from build123d import *

# Parameters (mm, degrees)
BOSS_EXTRUDE1_DEPTH = 6
SKETCH3_R           = 2
CUT_EXTRUDE1_DEPTH  = 5


with BuildPart() as part:
    # Sketch1 → Boss-Extrude1 (new body)
    with BuildSketch(Plane(origin=(0, 0, 0), x_dir=(1, 0, 0), z_dir=(0, 1, 0))):
        with BuildLine():
            Line((-1, 2.291287847), (-1, 4.291287847))
            Line((-1, 4.291287847), (1, 4.291287847))
            Line((1, 4.291287847), (1, 2.291287847))
            ThreePointArc((1, 2.291287847), (2.5, 0), (1, -2.291287847))
            Line((1, -2.291287847), (1, -4.291287847))
            Line((1, -4.291287847), (-1, -4.291287847))
            Line((-1, -4.291287847), (-1, -2.291287847))
            ThreePointArc((-1, -2.291287847), (-2.5, 0), (-1, 2.291287847))
        make_face()
    extrude(amount=BOSS_EXTRUDE1_DEPTH)

    # Sketch3 → Cut-Extrude1 (cut)
    with BuildSketch(Plane.XZ):
        with Locations(Location((0, 0, 0), (0, 0, 270))):
            Circle(SKETCH3_R)
    extrude(amount=-CUT_EXTRUDE1_DEPTH, mode=Mode.SUBTRACT)


solid = part.part
The model under review builds one solid part; all positions refer to its coordinate system, in mm. A direction names the side the tool comes from. Give positions to 0.01 mm unless a question says otherwise; leave off trailing zeros. Loops run counter-clockwise (first coordinate to the right, second up) from the corner with the lowest first, then second, coordinate; pieces in that order, holes last. Notation, with made-up numbers: (38, -5) -> (90, -5) arc R22 cw to (90, 21) -> close; hole circle Ø10 at (-24, 26). An arc over 180 degrees is marked (long way). Answer as a JSON object with one key per item and string values. Group by question number.
Q1. Insertion check: pin 1 (0.6 mm diameter, centred on y = 2.5, z = 3, fed in from -X); pin 2 (2 mm diameter, centred on y = 1, z = 2, fed in from -X); pin 3 (1.6 mm diameter, centred on y = 3, z = 3, fed in from +X). Each pin has a flat end and moves straight along its axis. Give the tip position at first contact, or say it passes through.
Q2. Wall thickness on line 1 along Y through (x, z) = (1.1, 1); line 2 along X through (y, z) = (4.75, 0.25); line 3 along X through (y, z) = (4.6, -1.5): over which ranges is each line inside the solid? List them lowest first.
Q3. Take a section at A-A (y = 3.8). Write out the cut boundary in (x, z), plus the area to 3 significant figures.
Q4. Tool access review of faces 1 (the flat face through (1, 3, 3)), 2 (the flat face through (-1, 3, 3)), 3 (the flat face through (-1, 3, -3)): name each direction out of +Z, -Z, +X, -X, +Y, -Y from which nothing blocks a thin tool from reaching the whole face with its end or side.
Q5. Draft analysis for pull direction Z (two halves, no side actions). For faces 4 (the flat face through (0, 5, 0)), 5 (the flat face through (0, 3, -4.291)), 6 (the flat face through (0, 6, 0)), 7 (the cylindrical face through (-2, 2, 0)), state which applies: pulls with the +Z half, pulls with the -Z half, needs draft (parallel to the pull), parting line crosses it, or undercut.
Q6. Take a section at C-C (x = 1.55). Write out the cut boundary in (y, z), plus the area to 3 significant figures.
Q7. Take a section at B-B (z = 0). Write out the cut boundary in (x, y), plus the area to 3 significant figures.
Q8. Take a section at D-D (z = 3). Write out the cut boundary in (x, y).
Answer below:
{
 "1": {"pin 1": "stops at x = -1", "pin 2": "stops at x = -2.29", "pin 3": "stops at x = 1.19"},
 "2": {"line 1": "y = 5 to 6", "line 2": "x = -2.49 to -1.98, 1.98 to 2.49", "line 3": "x = -2 to -1.32, 1.32 to 2"},
 "3": {"outline": "(-1, -4.29) -> (1, -4.29) -> (1, -2.29) arc R2.5 ccw to (1, 2.29) -> (1, 4.29) -> (-1, 4.29) -> (-1, 2.29) arc R2.5 ccw to (-1, -2.29) -> close; hole circle Ø4 at (0, 0)", "area": "14.5 mm2"},
 "4": {"face 1": "+Z, +X, +Y, -Y", "face 2": "+Z, -X, +Y, -Y", "face 3": "-Z, -X, +Y, -Y"},
 "5": {"face 4": "undercut", "face 5": "pulls with the -Z half", "face 6": "needs draft", "face 7": "undercut"},
 "6": {"outline": "(0, -1.96) -> (6, -1.96) -> (6, 1.96) -> (0, 1.96) -> (0, 1.26) -> (5, 1.26) -> (5, -1.26) -> (0, -1.26) -> close", "area": "10.9 mm2"},
 "7": {"outline": "(-2.5, 0) -> (-2, 0) -> (-2, 5) -> (2, 5) -> (2, 0) -> (2.5, 0) -> (2.5, 6) -> (-2.5, 6) -> close", "area": "10.0 mm2"},
 "8": {"outline": "(-1, 0) -> (1, 0) -> (1, 6) -> (-1, 6) -> close"}
}
